from build123d import *

# Parameters (mm, degrees)
F0_W      = 64
F0_H      = 1.5
F1_DEPTH  = 23
F0_H_2    = 83
F2_DEPTH  = 1.5
F3_W      = 10
F3_H      = 10
F4_DEPTH  = 5
F5_W      = 10
F5_H      = 5
F6_DEPTH  = 25
F7_W      = 10
F7_H      = 5
F8_DEPTH  = 5
F10_DEPTH = 47.7


with BuildPart() as f1:
    # F0 (on Top) → F1 (new body)
    with BuildSketch(Plane.XY):
        Polygon((-32, 48.42079), (-33.5, 48.42079), (-33.5, -36.07921), (-32, -36.07921), (-32, -34.57921), align=None)
        with Locations((0, -35.32921)):
            Rectangle(F0_W, F0_H)
        Polygon((33.5, 48.42079), (32, 48.42079), (32, -34.57921), (32, -36.07921), (33.5, -36.07921), align=None)
    extrude(amount=F1_DEPTH)

    # F0 (on Top) → F2 (join)
    with BuildSketch(Plane.XY):
        Polygon((-32, 48.42079), (-33.5, 48.42079), (-33.5, -36.07921), (-32, -36.07921), (-32, -34.57921), align=None)
        with Locations((0, 6.92079)):
            Rectangle(F0_W, F0_H_2)
        Polygon((33.5, 48.42079), (32, 48.42079), (32, -34.57921), (32, -36.07921), (33.5, -36.07921), align=None)
        with Locations((0, -35.32921)):
            Rectangle(F0_W, F0_H)
    extrude(amount=F2_DEPTH)

    # F3 (on face) → F4 (join)
    with BuildSketch(Plane(origin=(0, 0, 0), x_dir=(1, 0, 0), z_dir=(0, 0, -1))):
        with Locations((16.75, -43.42079)):
            Rectangle(F3_W, F3_H)
        with Locations((-16.75, -43.42079)):
            Rectangle(F3_W, F3_H)
    extrude(amount=F4_DEPTH)

    # F5 (on face) → F6 (join)
    with BuildSketch(Plane(origin=(0, 48.42079, 0), x_dir=(-1, 0, 0), z_dir=(0, 1, 0))):
        with Locations((-16.75, -2.5)):
            Rectangle(F5_W, F5_H)
        with Locations((16.75, -2.5)):
            Rectangle(F5_W, F5_H)
    extrude(amount=F6_DEPTH)

    # F7 (on face) → F8 (join)
    with BuildSketch(Plane.XY):
        with Locations((16.75, 70.92079)):
            Rectangle(F7_W, F7_H)
        with Locations((-16.75, 70.92079)):
            Rectangle(F7_W, F7_H)
    extrude(amount=F8_DEPTH)

    # F9 (on face) → F10 (cut)
    with BuildSketch(Plane.YZ.offset(21.75)):
        Polygon((73.42079, 5), (68.42079, 5), (68.42079, 4.5), (73.42079, 0), align=None)
    extrude(amount=-F10_DEPTH, mode=Mode.SUBTRACT)


with BuildPart() as f11_1:
    # F11: copy of F1
    add(f1.part)


solid = f11_1.part
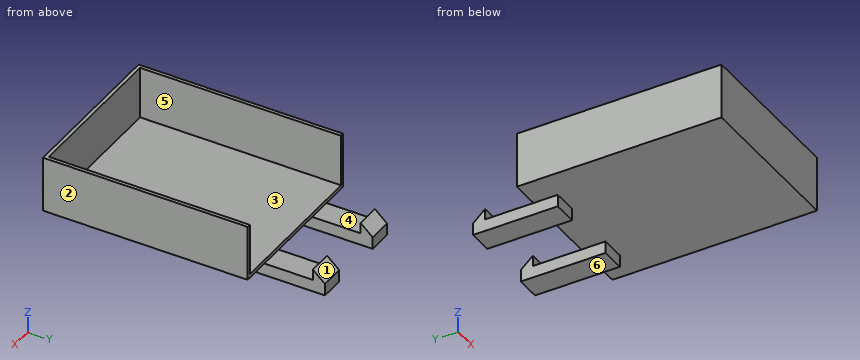
The listing builds one solid part. Answer for the finished solid, in the listing's coordinates (mm). Face numbers are marked on the shaded views. A direction names the side the tool comes from. Round coordinates to 2 decimals unless told otherwise and drop trailing zeros. Order: outer loops, then holes, each group sorted by start corner. A loop starts at its lowest first (then second) coordinate and runs counter-clockwise, first axis right, second up. Notation, with made-up numbers: (-33, 72) -> (-28, 72) arc R19 ccw to (-28, 100) -> close; hole circle Ø9 at (45, 25). An arc over 180 degrees is marked (long way). Write each question's results on one line, items separated by ' | '. Start each with the question number.
Q1. Straight lines are drawn through the part: probe 1 along X at (y, z) = (10.5, 5); probe 2 along Z at (x, y) = (-15.5, 38.5); probe 3 along Y at (x, z) = (26, 12.25). For each, find the intervals that lie inside material, in ascending order. Write a range as from..to.
Q2. Which of the six approach directions +Z, -Z, +X, -X, +Y, -Y give full straight-line access (tool end or side, diameter ignored) to the marked faces 4, 5 and 6?
Q3. Each of these flat-tipped pins is pushed along its axis until it touches: pin 1 (5 mm diameter, centred on x = 16.5, y = 56.5, fed in from +Z); pin 2 (8 mm diameter, centred on x = -9, z = 12.5, fed in from +Y); pin 3 (10 mm diameter, centred on x = 26.5, y = 9, fed in from +Z). Where does it stop, or does it pass through?
Q4. Find section B-B (x = 9). Determine the outline of the cut face in (y, z).
Q5. Find section A-A (y = 53.5). Determine the outline of the cut face in (x, z), then the cut area to 3 significant figures.
Q6. The mould has two halves that part along X. Classify the marked faces 1, 2 and 3: pulls with the +X half, pulls with the -X half, needs draft (parallel to the pull), parting line crosses it, or undercut.
Q7. Find section D-D (z = 3). Determine the outline of the cut face in (x, y).
Q8. Find section C-C (y = 27). Determine the outline of the cut face in (x, z), then the cut area to 3 significant figures.
Worked answers:
1) probe 1: x = -33.5..-32, 32..33.5 | probe 2: z = -5..1.5 | probe 3: y = -36.08..-34.58
2) face 4: +Z, +X, -X | face 5: +Z, +Y | face 6: -Z, +X, -X, +Y, -Y
3) pin 1: stops at z = 0 | pin 2: stops at y = -34.58 | pin 3: stops at z = 1.5
4) outline: (-36.08, 0) -> (48.42, 0) -> (48.42, 1.5) -> (-34.58, 1.5) -> (-34.58, 23) -> (-36.08, 23) -> close
5) outline: (-21.75, -5) -> (-11.75, -5) -> (-11.75, 0) -> (-21.75, 0) -> close; (11.75, -5) -> (21.75, -5) -> (21.75, 0) -> (11.75, 0) -> close | area: 100 mm2
6) face 1: needs draft | face 2: pulls with the +X half | face 3: undercut
7) outline: (-33.5, -36.08) -> (33.5, -36.08) -> (33.5, 48.42) -> (32, 48.42) -> (32, -34.58) -> (-32, -34.58) -> (-32, 48.42) -> (-33.5, 48.42) -> close; (-21.75, 68.42) -> (-11.75, 68.42) -> (-11.75, 70.09) -> (-21.75, 70.09) -> close; (11.75, 68.42) -> (21.75, 68.42) -> (21.75, 70.09) -> (11.75, 70.09) -> close
8) outline: (-33.5, 0) -> (33.5, 0) -> (33.5, 23) -> (32, 23) -> (32, 1.5) -> (-32, 1.5) -> (-32, 23) -> (-33.5, 23) -> close | area: 165 mm2
